from build123d import *

# Parameters (mm, degrees)
F0_W     = 57.15
F0_H     = 76.2
F2_DEPTH = 6.35
F1_W     = 50.8
F1_H     = 50.8
F1_W_2   = 45.466
F1_H_2   = 45.466
F3_DEPTH = 38.1
F4_START = -33.655
F4_DEPTH = 4.445


# Not quite as in the source:
# - a feature names something its author has since deleted; it is built from what else it names


with BuildPart() as f2:
    # F0 (on Front) → F2 (new body)
    with BuildSketch(Plane.XZ):
        Rectangle(F0_W, F0_H)
    extrude(amount=-F2_DEPTH)

    # F1 (on Top) → F3 (join, symmetric)
    with BuildSketch(Plane.XY):
        with Locations((0, -25.4)):
            Rectangle(F1_W, F1_H)
        with Locations((0, -25.4)):
            Rectangle(F1_W_2, F1_H_2, mode=Mode.SUBTRACT)
    extrude(amount=F3_DEPTH, both=True)

    # F1 (on Top) → F4 (join)
    with BuildSketch(Plane.XY.offset(F4_START)):
        with Locations((0, -25.4)):
            Rectangle(F1_W_2, F1_H_2)
    extrude(amount=-F4_DEPTH)


solid = f2.part
Geometry: final body of the model. Coordinates: model frame, mm. A direction names the side the tool comes from. Round coordinates to 2 decimals unless told otherwise and drop trailing zeros. Order: outer loops, then holes, each group sorted by start corner. A loop starts at its lowest first (then second) coordinate and runs counter-clockwise, first axis right, second up. Notation, with made-up numbers: (17, 51) -> (35, 51) arc R21 cw to (35, 89) -> close; hole circle Ø1 at (40.5, 71). An arc over 180 degrees is marked (long way). Put each result on its own line as item: value. Start each with the question number.
Q1. Section C-C on y = -25. Return the cut outline in (x, z) (3 decimals).
Q2. Section B-B on z = 32. Return the cut outline in (x, y) (3 decimals), and give its area (3 significant figures).
Q3. Section A-A on x = 12. Return the cut outline in (y, z) (3 decimals).
Q4. Pull-direction query (X, two-part tool) for faces 1 (the flat face through (25.4, -26, 1)), 2 (the flat face through (-22.733, -26, 3)), 3 (the flat face through (0, -48.133, 3)), 4 (the flat face through (2, -1, 38.1)); classes: +X half, -X half, draft (parallel to the pull), parting line (faces both ways), or undercut.
Q5. Reachability of faces 5 (the flat face through (27, 0, 1)), 6 (the flat face through (0, -23, -38.1)), 7 (the flat face through (0, -50.8, 1)), 8 (the flat face through (-27, 0, 1)), 9 (the flat face through (22.733, -26, 3)) from +Z, -Z, +X, -X, +Y, -Y: full face, straight path, thin tool, end or side. Return the list, or none.
Q6. Line query: probe 1 along Y at (x, z) = (18.5, -25.5); probe 2 along X at (y, z) = (-45.5, -30); probe 3 along Z at (x, y) = (-22.5, -27) (3 decimals). Output: solid intervals per line, ascending.
Q7. First-contact query: pin 1 (2.5 mm diameter, centred on x = -27.5, z = 15, fed in from -Y); pin 2 (2 mm diameter, centred on y = -31.5, z = 29, fed in from -X); pin 3 (8 mm diameter, centred on y = -2.5, z = -17.5, fed in from +X) (3 decimals); pin 4 (22.5 mm diameter, centred on x = 10, y = -33.5, fed in from +Z) (3 decimals). Flat tips, straight axial feed; report the tip coordinate or a pass-through.
Ans:
1. outline: (-25.4, -38.1) -> (25.4, -38.1) -> (25.4, 38.1) -> (22.733, 38.1) -> (22.733, -33.655) -> (-22.733, -33.655) -> (-22.733, 38.1) -> (-25.4, 38.1) -> close
2. outline: (-28.575, 0) -> (-25.4, 0) -> (-25.4, -50.8) -> (25.4, -50.8) -> (25.4, 0) -> (28.575, 0) -> (28.575, 6.35) -> (-28.575, 6.35) -> close; hole (-22.733, -48.133) -> (22.733, -48.133) -> (22.733, -2.667) -> (-22.733, -2.667) -> close
2. area: 876 mm2
3. outline: (-50.8, -38.1) -> (6.35, -38.1) -> (6.35, 38.1) -> (-2.667, 38.1) -> (-2.667, -33.655) -> (-48.133, -33.655) -> (-48.133, 38.1) -> (-50.8, 38.1) -> close
4. face 1: +X half
4. face 2: undercut
4. face 3: undercut
4. face 4: draft
5. face 5: +Z, -Z, +X, -Y
5. face 6: -Z, +X, -X, +Y, -Y
5. face 7: +Z, -Z, +X, -X, -Y
5. face 8: +Z, -Z, -X, -Y
5. face 9: +Z
6. probe 1: y = -50.8 to -48.13, -2.67 to 6.35
6. probe 2: x = -25.4 to -22.73, 22.73 to 25.4
6. probe 3: z = -38.1 to -33.655
7. pin 1: stops at y = 0
7. pin 2: stops at x = -25.4
7. pin 3: stops at x = 28.575
7. pin 4: stops at z = -33.655
